Here's how the part is built. I have some questions about the finished solid (model axes, mm). Coordinates: 2 decimals unless noted, no trailing zeros. Order: outer loops, then holes, each group sorted by start corner. A loop starts at its lowest first (then second) coordinate and runs counter-clockwise, first axis right, second up. Notation, with made-up numbers: (59.25, 77) - (115.25, 77) arc R13 cw to (115.25, 98) - close; hole circle Ø3 at (-21, -5.75). An arc over 180 degrees is marked (long way). Answer as CSV lines item,"result". Start each with the question number.
Q1. Suppose I cut it at A-A (x = 12). Please give me the cut outline in (y, z) (3 decimals), then the cut area to 3 significant figures.
Q2. I need wall thicknesses on line 1 (Y direction, x = -4, z = 6); line 2 (Y direction, x = 11.5, z = 4.5); line 3 (X direction, y = 0.5, z = 1.25). Which ranges of each line are inside material? Lowest first, please.
Q3. For pin 1 Ø1.2 at (x, y) = (12.1, -14.7) entering from -Z, with a flat end and sliding along its axis, tell me the tip position at first contact or that it passes through.
Q4. Suppose I cut it at B-B (z = 1). Count the separate pieces of the cut face and the enclosed holes in it, then the cut area to 3 significant figures.
Autodesk Inventor part; units mm, degrees
ref_plane "YZ Plane" through (0, 0, 0) normal (1, 0, 0) x (0, 1, 0)
ref_plane "XZ Plane" through (0, 0, 0) normal (0, 1, 0) x (-1, 0, 0)
ref_plane "XY Plane" through (0, 0, 0) normal (0, 0, 1) x (1, 0, 0)
sketch "Sketch1" plane through (0, 0, 0) normal (0, 0, 1) x (1, 0, 0)
  line L0 (-15.9035, 8.2993) -> (24.0965, 8.2993)
  line L1 (24.0965, 8.2993) -> (24.0965, -21.7007)
  line L2 (24.0965, -21.7007) -> (-15.9035, -21.7007)
  line L3 (-15.9035, -21.7007) -> (-15.9035, 8.2993)
  point P0 (0, 0)
  dimension "d0" = 40
  dimension "d1" = 30
extrude "Extrusion1" add sketch "Sketch1" along normal blind 2
sketch "Sketch2" plane through (0, 0, 2) normal (0, 0, 1) x (1, 0, 0)
  line L0 (-15.9035, -21.7007) -> (-15.9035, 8.2993)
  line L1 (24.0965, -21.7007) -> (-15.9035, -21.7007)
  line L2 (-15.9035, -6.7007) -> (4.0965, -6.7007)
  line L3 (4.0965, -6.7007) -> (4.0965, -14.7007)
  line L4 (4.0965, -14.7007) -> (-3.9035, -14.7007)
  line L5 (-3.9035, -14.7007) -> (-3.9035, 1.2993)
  line L6 (-3.9035, 1.2993) -> (12.0965, 1.2993)
  line L7 (12.0965, 1.2993) -> (12.0965, -14.7007)
  circle A0 centre (12.0965, -6.7007) radius 1
  circle A1 centre (12.0965, 1.2993) radius 1
  circle A2 centre (4.0965, 1.2993) radius 1
  circle A3 centre (-3.9035, 1.2993) radius 1
  circle A4 centre (-3.9035, -6.7007) radius 1
  circle A5 centre (-3.9035, -14.7007) radius 1
  circle A6 centre (4.0965, -14.7007) radius 1
  circle A7 centre (12.0965, -14.7007) radius 1
  point P0 (0, 0)
  dimension "d4" = 8
  dimension "d5" = 8
  dimension "d6" = 16
  dimension "d7" = 16
  dimension "d8" = 16
  dimension "d9" = 2
extrude "Extrusion2" cut sketch "Sketch2" against normal blind 2 contours A7 | A0 L7 | L7 A0 | A1 L7 L6 | L6 L7 A1 | A2 L6 | L6 A2 | A3 L6 L5 | L5 L6 A3 | A4 L5 L2 | L2 L5 A4 | L5 A4 L2 | L2 A4 L5 | A6 L4 L3 | L3 L4 A6 | A5 L4 L5 | L5 L4 A5
sketch "Sketch3" plane through (-15.9035, -21.7007, 0) normal (0, -1, 0) x (1, 0, 0)
  line L0 (40, 2) -> (0, 2)
  line L1 (0, 0) -> (0, 2)
  line L2 (40, 0) -> (0, 0)
  line L3 (40, 0) -> (40, 2)
  point P0 (15.9035, 0)
extrude "Extrusion3" add sketch "Sketch3" along normal blind 1
sketch "Sketch4" plane through (-15.9035, 8.2993, 0) normal (0, 1, 0) x (1, 0, 0)
  line L0 (0, -2) -> (40, -2)
  line L1 (40, 0) -> (40, -2)
  line L2 (0, 0) -> (40, 0)
  line L3 (0, 0) -> (0, -2)
  point P0 (15.9035, 0)
extrude "Extrusion4" add sketch "Sketch4" along normal blind 1
sketch "Sketch5" plane through (0, 0, 2) normal (0, 0, 1) x (1, 0, 0)
  circle A0 centre (12.0965, -14.7007) radius 1
  circle A1 centre (4.0965, -14.7007) radius 1
  circle A2 centre (-3.9035, -14.7007) radius 1
  circle A3 centre (-3.9035, -6.7007) radius 1
  circle A4 centre (-3.9035, 1.2993) radius 1
  circle A5 centre (4.0965, 1.2993) radius 1
  circle A6 centre (12.0965, 1.2993) radius 1
  circle A7 centre (12.0965, -6.7007) radius 1
  line L0 (24.0965, 9.2993) -> (24.0965, -22.7007)
  line L1 (24.0965, 9.2993) -> (-15.9035, 9.2993)
  line L2 (-15.9035, -22.7007) -> (-15.9035, 9.2993)
  line L3 (-15.9035, -22.7007) -> (24.0965, -22.7007)
  point P0 (0, 0)
extrude "Extrusion5" add sketch "Sketch5" along normal blind 9.525
sketch "Sketch6" plane through (0, 0, 0) normal (0, 0, -1) x (-1, 0, 0)
  circle A0 centre (-12.0965, -14.7007) radius 1
  circle A1 centre (-4.0965, -14.7007) radius 1
  circle A2 centre (3.9035, -14.7007) radius 1
  circle A3 centre (3.9035, -6.7007) radius 1
  circle A4 centre (3.9035, 1.2993) radius 1
  circle A5 centre (-4.0965, 1.2993) radius 1
  circle A6 centre (-12.0965, 1.2993) radius 1
  circle A7 centre (-12.0965, -6.7007) radius 1
  line L0 (-24.0965, 9.2993) -> (-24.0965, -22.7007)
  line L1 (-24.0965, -22.7007) -> (15.9035, -22.7007)
  line L2 (15.9035, -22.7007) -> (15.9035, 9.2993)
  line L3 (15.9035, 9.2993) -> (-24.0965, 9.2993)
  point P0 (0, 0)
extrude "Extrusion6" add sketch "Sketch6" along normal blind 1.1684
sketch "Sketch7" plane through (-15.9035, -22.7007, 0) normal (0, -1, 0) x (1, 0, 0)
  line L0 (40, 11.525) -> (0, 11.525)
  line L1 (0, -1.1684) -> (1, -1.1684)
  line L2 (1, -1.1684) -> (1, 11.525)
  line L3 (1, 11.525) -> (0, 11.525)
  line L4 (0, 11.525) -> (0, -1.1684)
  point P0 (15.9035, 0)
  dimension "d20" = 1
extrude "Extrusion7" cut sketch "Sketch7" against normal blind 50.8
properties part number "hconnector"
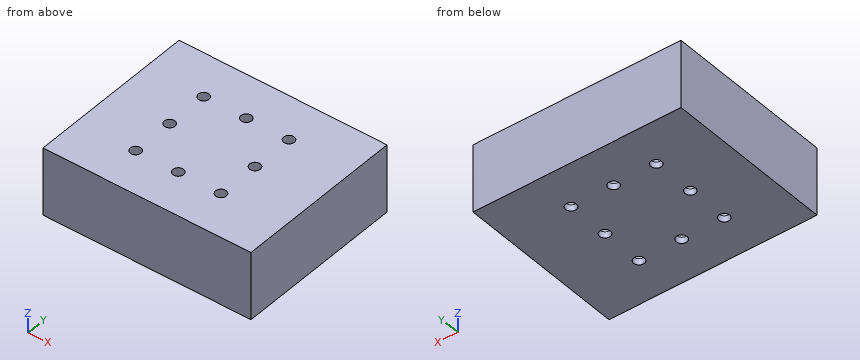
Here are the results:
1,outline,"(-22.701, -1.168) - (-15.696, -1.168) - (-15.696, 11.525) - (-22.701, 11.525) - close; (-13.705, -1.168) - (-7.696, -1.168) - (-7.696, 11.525) - (-13.705, 11.525) - close; (-5.705, -1.168) - (0.304, -1.168) - (0.304, 11.525) - (-5.705, 11.525) - close; (2.295, -1.168) - (9.299, -1.168) - (9.299, 11.525) - (2.295, 11.525) - close"
1,area,"330 mm²"
2,line 1,"y = -22.7 to -15.7, -13.71 to -7.7, -5.71 to 0.3, 2.29 to 9.3"
2,line 2,"y = -22.7 to -15.5, -13.9 to -7.5, -5.9 to 0.5, 2.1 to 9.3"
2,line 3,"x = -14.9 to -4.5, -3.3 to 3.5, 4.7 to 11.5, 12.7 to 24.1"
3,pin 1,"passes through"
4,separate pieces,"1"
4,enclosed holes,"8"
4,area,"1,220 mm²"
